Part model, mm, in its own coordinate system. Face numbers are marked on the shaded views. A direction names the side the tool comes from. Give positions to 0.01 mm unless a question says otherwise; leave off trailing zeros. Loops run counter-clockwise (first coordinate to the right, second up) from the corner with the lowest first, then second, coordinate; pieces in that order, holes last. Notation, with made-up numbers: (68.25, -5) -> (109.25, -5) arc R6 ccw to (109.25, 1) -> close; hole circle Ø11 at (61.5, 60). An arc over 180 degrees is marked (long way). One line per question, with ' | ' between items.
```python
from build123d import *

# Parameters (mm, degrees)
BOSS_EXTRUDE1_DEPTH = 20
FILLET1_R           = 10
SKETCH2_R           = 5
CUT_EXTRUDE1_DEPTH  = 40


with BuildPart() as part:
    # Sketch1 → Boss-Extrude1 (new, symmetric)
    with BuildSketch(Plane.XY):
        with BuildLine():
            Line((-70, 15), (-47.696960071, 15))
            ThreePointArc((-47.696960071, 15), (50, 0), (-47.696960071, -15))
            Line((-47.696960071, -15), (-70, -15))
            Line((-70, -15), (-70, -11))
            Line((-70, -11), (-44.665422868, -11))
            ThreePointArc((-44.665422868, -11), (46, 0), (-44.665422868, 11))
            Line((-44.665422868, 11), (-70, 11))
            Line((-70, 11), (-70, 15))
        make_face()
    extrude(amount=BOSS_EXTRUDE1_DEPTH, both=True)

    # Fillet1
    fillet1_edges = [part.edges().sort_by_distance(p)[0] for p in [
        (-70, -13, -20),
        (-70, 13, 20),
        (-70, -13, 20),
        (-70, 13, -20),
    ]]
    fillet(fillet1_edges, radius=FILLET1_R)

    # Sketch2 → Cut-Extrude1 (cut)
    with BuildSketch(Plane(origin=(0, 15, 0), x_dir=(1, 0, 0), z_dir=(0, 1, 0))):
        with Locations(Location((-60, 0, 0), (0, 0, 270))):
            Circle(SKETCH2_R)
    extrude(amount=-CUT_EXTRUDE1_DEPTH, mode=Mode.SUBTRACT)


solid = part.part
```
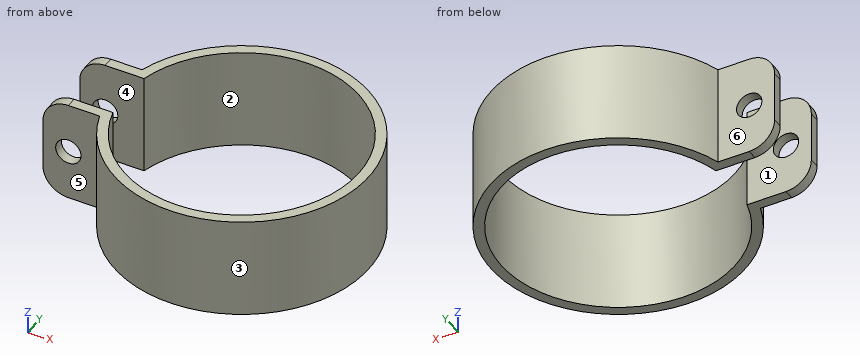
1) Drill centre lines: line 1 (Y direction, x = -61, z = 16.5); line 2 (X direction, y = 13, z = 0); line 3 (Y direction, x = 0, z = 5). Where is each one in solid material? Low to high.
Found:
line 1: -15 to -11, 11 to 15 | line 2: -70 to -65, -55 to -44.12, 44.12 to 48.28 | line 3: -50 to -46, 46 to 50
2) Pin check, flat tips, straight feed: P1, Ø12, axis at x = -54.5, z = 10.5, coming from the -Y side; P2, Ø10, axis at x = 25, z = 11.5, coming from the +Y side; P3, Ø7.5, axis at x = -54, z = 3.5, coming from the +Y side. Stop position of each tip, or through.
Found:
P1: y = -15 | P2: y = 45.83 | P3: y = 15
3) Saw through at A-A (x = 0). Give the cut face in (y, z).
Found:
outline: (-50, -20) -> (-46, -20) -> (-46, 20) -> (-50, 20) -> close; (46, -20) -> (50, -20) -> (50, 20) -> (46, 20) -> close
4) Saw through at B-B (z = -3). Give the cut face in (x, y).
Found:
outline: (-70, -15) -> (-64, -15) -> (-64, -11) -> (-70, -11) -> close; (-70, 11) -> (-64, 11) -> (-64, 15) -> (-70, 15) -> close; (-56, -15) -> (-47.7, -15) arc R50 ccw (long way) to (-47.7, 15) -> (-56, 15) -> (-56, 11) -> (-44.67, 11) arc R46 cw (long way) to (-44.67, -11) -> (-56, -11) -> close
5) Pull direction X, two halves, no side cores. Call the marked faces 1, 2 and 3: pulls with the +X half, pulls with the -X half, needs draft (parallel to the pull), parting line crosses it, or undercut.
Found:
face 1: needs draft | face 2: undercut | face 3: parting line crosses it
6) Saw through at C-C (y = 21). Give the cut face in (x, z), and give its area (3 significant figures).
Found:
outline: (-45.38, -20) -> (-40.93, -20) -> (-40.93, 20) -> (-45.38, 20) -> close; (40.93, -20) -> (45.38, -20) -> (45.38, 20) -> (40.93, 20) -> close | area: 356 mm2
7) Saw through at D-D (z = 14.5). Give the cut face in (x, y).
Found:
outline: (-68.93, -15) -> (-47.7, -15) arc R50 ccw (long way) to (-47.7, 15) -> (-68.93, 15) -> (-68.93, 11) -> (-44.67, 11) arc R46 cw (long way) to (-44.67, -11) -> (-68.93, -11) -> close
8) Tool access for the marked faces 4, 5 and 6: list every direction of +Z, -Z, +X, -X, +Y, -Y with a clear straight run to the whole face (end or side of a thin tool).
Found:
face 4: +Z, -Z, -X | face 5: +Z, -Z, -X, -Y | face 6: +Z, -Z, -X, +Y
